Design review of the part built by this model. Coordinates are the model's own, in mm. A direction names the side the tool comes from. Coordinates: 2 decimals unless noted, no trailing zeros. Order: outer loops, then holes, each group sorted by start corner. A loop starts at its lowest first (then second) coordinate and runs counter-clockwise, first axis right, second up. Notation, with made-up numbers: M 73,-16 L 107,-16 A10 cw 107,-5 Z; hole C -39.75,22 d3. An arc over 180 degrees is marked long. Answer in a Markdown table with one row per item.
from build123d import *

# Parameters (mm, degrees)
SKETCH_1_W          = 98
SKETCH_1_H          = 95
EXTRUDE_1_DEPTH     = 1
SKETCH_2_W          = 78
SKETCH_2_H          = 85
EXTRUDE_2_DEPTH     = 20
CUT_EXTRUDE_1_DEPTH = 100
CUT_EXTRUDE_2_DEPTH = 5
SKETCH_5_W          = 9
SKETCH_5_H          = 12
EXTRUDE_3_DEPTH     = 5
SKETCH_6_W          = 11.2
SKETCH_6_H          = 4.6
SKETCH_6_W_2        = 10.2
SKETCH_6_H_2        = 1.749108458
CUT_EXTRUDE_4_DEPTH = 8
CUT_EXTRUDE_5_DEPTH = 0.5


with BuildPart() as part:
    # 스케치1 → 보스-돌출1 (new body)
    with BuildSketch(Plane(origin=(0, 0, 0), x_dir=(1, 0, 0), z_dir=(0, 1, 0))):
        Rectangle(SKETCH_1_W, SKETCH_1_H)
    extrude(amount=EXTRUDE_1_DEPTH)

    # 스케치2 → 보스-돌출2 (add)
    with BuildSketch(Plane(origin=(0, 1, 0), x_dir=(1, 0, 0), z_dir=(0, 1, 0))):
        with Locations((5, 0)):
            Rectangle(SKETCH_2_W, SKETCH_2_H)
    extrude(amount=EXTRUDE_2_DEPTH)

    # 스케치4 → 컷-돌출1 (cut)
    with BuildSketch(Plane(origin=(44, 0, 0), x_dir=(0, 0, -1), z_dir=(1, 0, 0))):
        with BuildLine():
            Line((-42.5, 1), (-41.5, 1))
            Line((-41.5, 1), (-41.5, 12.254740451))
            Line((-41.5, 12.254740451), (-40.591554577, 12.962724137))
            ThreePointArc((-40.591554577, 12.962724137), (-37.80324019, 18.684012014), (-31.875, 21))
            Line((-31.875, 21), (-42.5, 21))
            Line((-42.5, 21), (-42.5, 1))
        make_face()
        with BuildLine():
            Line((-22.25, 12.254740451), (-22.25, 1))
            Line((-22.25, 1), (-20.25, 1))
            Line((-20.25, 1), (-20.25, 12.254740451))
            Line((-20.25, 12.254740451), (-19.341554577, 12.962724137))
            ThreePointArc((-19.341554577, 12.962724137), (-16.553240185, 18.684012019), (-10.624999986, 21))
            Line((-10.624999986, 21), (-31.875, 21))
            ThreePointArc((-31.875, 21), (-25.94675981, 18.684012014), (-23.158445423, 12.962724137))
            Line((-23.158445423, 12.962724137), (-22.25, 12.254740451))
        make_face()
        with BuildLine():
            Line((-1, 12.254740451), (-1, 1))
            Line((-1, 1), (1, 1))
            Line((1, 1), (1, 12.254740451))
            Line((1, 12.254740451), (1.908445423, 12.962724137))
            ThreePointArc((1.908445423, 12.962724137), (4.696759796, 18.684012001), (10.62499996, 21))
            Line((10.62499996, 21), (-10.624999986, 21))
            ThreePointArc((-10.624999986, 21), (-4.696759805, 18.68401201), (-1.908445423, 12.962724137))
            Line((-1.908445423, 12.962724137), (-1, 12.254740451))
        make_face()
        with BuildLine():
            Line((20.25, 12.254740451), (20.25, 1))
            Line((20.25, 1), (22.25, 1))
            Line((22.25, 1), (22.25, 12.254740451))
            Line((22.25, 12.254740451), (23.158445423, 12.962724137))
            ThreePointArc((23.158445423, 12.962724137), (25.94675981, 18.684012014), (31.875, 21))
            Line((31.875, 21), (10.62499996, 21))
            ThreePointArc((10.62499996, 21), (16.553240175, 18.684012028), (19.341554577, 12.962724137))
            Line((19.341554577, 12.962724137), (20.25, 12.254740451))
        make_face()
        with BuildLine():
            Line((42.5, 21), (31.875, 21))
            ThreePointArc((31.875, 21), (37.80324019, 18.684012014), (40.591554577, 12.962724137))
            Line((40.591554577, 12.962724137), (41.5, 12.254740451))
            Line((41.5, 12.254740451), (41.5, 1))
            Line((41.5, 1), (42.5, 1))
            Line((42.5, 1), (42.5, 21))
        make_face()
    extrude(amount=-CUT_EXTRUDE_1_DEPTH, mode=Mode.SUBTRACT)

    # 스케치4<3> → 컷-돌출2 (cut)
    with BuildSketch(Plane(origin=(44, 0, 0), x_dir=(0, 0, -1), z_dir=(1, 0, 0))):
        with BuildLine():
            ThreePointArc((-23.158445423, 12.962724137), (-31.875, 21), (-40.591554577, 12.962724137))
            Line((-40.591554577, 12.962724137), (-36.685, 16.007240451))
            Line((-36.685, 16.007240451), (-27.065, 16.007240451))
            Line((-27.065, 16.007240451), (-23.158445423, 12.962724137))
        make_face()
        with BuildLine():
            Line((-5.815, 16.007240451), (-1.908445423, 12.962724137))
            ThreePointArc((-1.908445423, 12.962724137), (-10.625, 21), (-19.341554577, 12.962724137))
            Line((-19.341554577, 12.962724137), (-15.435, 16.007240451))
            Line((-15.435, 16.007240451), (-5.815, 16.007240451))
        make_face()
        with BuildLine():
            Line((15.435, 16.007240451), (19.341554577, 12.962724137))
            ThreePointArc((19.341554577, 12.962724137), (10.625, 21), (1.908445423, 12.962724137))
            Line((1.908445423, 12.962724137), (5.815, 16.007240451))
            Line((5.815, 16.007240451), (15.435, 16.007240451))
        make_face()
        with BuildLine():
            Line((36.685, 16.007240451), (40.591554577, 12.962724137))
            ThreePointArc((40.591554577, 12.962724137), (31.875, 21), (23.158445423, 12.962724137))
            Line((23.158445423, 12.962724137), (27.065, 16.007240451))
            Line((27.065, 16.007240451), (36.685, 16.007240451))
        make_face()
    extrude(amount=-CUT_EXTRUDE_2_DEPTH, mode=Mode.SUBTRACT)

    # 스케치5 → 보스-돌출3 (add)
    with BuildSketch(Plane(origin=(0, 1, 0), x_dir=(1, 0, 0), z_dir=(0, 1, 0))):
        with Locations((-44.5, 0)):
            Rectangle(SKETCH_5_W, SKETCH_5_H)
    extrude(amount=EXTRUDE_3_DEPTH)

    # 스케치6 → 컷-돌출4 (cut)
    with BuildSketch(Plane.ZY.offset(49)):
        with Locations((0, 3.3)):
            Rectangle(SKETCH_6_W, SKETCH_6_H)
        with Locations((0, 4.300145796)):
            Rectangle(SKETCH_6_W_2, SKETCH_6_H_2, mode=Mode.SUBTRACT)
    extrude(amount=-CUT_EXTRUDE_4_DEPTH, mode=Mode.SUBTRACT)

    # 스케치7 → 컷-돌출5 (cut)
    with BuildSketch(Plane(origin=(0, 6, 0), x_dir=(1, 0, 0), z_dir=(0, 1, 0))):
        Polygon((-42.731367286, 2.836850655), (-46.283445156, 2.836850655), (-47.255371975, 2.487236692), (-47.255371975, 1.305541495), (-46.33938339, 0.68322864), (-42.731367286, 0.68322864), (-42.731367286, 0.994385067), (-46.33938339, 0.994385067), (-46.960091467, 1.416087501), (-46.960091467, 2.396337061), (-46.33938339, 2.619613348), (-42.731367286, 2.619613348), align=None)
        Polygon((-42.731367286, -2.836850655), (-46.283445156, -2.836850655), (-47.255371975, -2.487236692), (-47.255371975, -1.305541495), (-46.33938339, -0.68322864), (-42.731367286, -0.68322864), (-42.731367286, -0.994385067), (-46.33938339, -0.994385067), (-46.960091467, -1.416087501), (-46.960091467, -2.396337061), (-46.33938339, -2.619613348), (-42.731367286, -2.619613348), align=None)
    extrude(amount=-CUT_EXTRUDE_5_DEPTH, mode=Mode.SUBTRACT)


solid = part.part
(1) Draft analysis for pull direction Y (two halves, no side actions). For faces 4 (the flat face through (-34, 11, 32)), 5 (the flat face through (42, 16.007, 32)), 6 (the flat face through (-45, 5.6, 0)), state which applies: pulls with the +Y half, pulls with the -Y half, needs draft (parallel to the pull), parting line crosses it, or undercut.
Return value:
| item | result |
|---|---|
| face 4 | needs draft |
| face 5 | pulls with the +Y half |
| face 6 | undercut |
(2) Insertion check: pin 1 Ø2.5 at (x, z) = (42.5, 11.5) entering from +Y; pin 2 Ø6 at (y, z) = (8, -28.5) entering from -X; pin 3 Ø1.5 at (x, y) = (33, 4) entering from -Z; pin 4 Ø3 at (x, z) = (-39, 13) entering from -Y. Each pin has a flat end and moves straight along its axis. Give the tip position at first contact, or say it passes through.
Return value:
| item | result |
|---|---|
| pin 1 | stops at y = 16.01 |
| pin 2 | stops at x = -34 |
| pin 3 | stops at z = -41.5 |
| pin 4 | stops at y = 0 |
(3) Add section C-C, the plane z = 30.5. Give the boundary of the cut face in (x, y).
Return value:
| item | result |
|---|---|
| outline | M -49,0 L 49,0 L 49,1 L 44,1 L 44,16.01 L 39,16.01 L 39,20.89 L -34,20.89 L -34,1 L -49,1 Z |
(4) For line 1 along Z through (x, y) = (-1.5, 4); line 2 along Z through (x, y) = (-42, 4.75); line 3 along Z through (x, y) = (16, 16.5), list the stretches that pass through material, from the lowest coordinate up. Write a range as from..to.
Return value:
| item | result |
|---|---|
| line 1 | z = -41.5..-22.25, -20.25..-1, 1..20.25, 22.25..41.5 |
| line 2 | z = -6..-5.6, -5.1..5.1, 5.6..6 |
| line 3 | z = -39.52..-24.23, -18.27..-2.98, 2.98..18.27, 24.23..39.52 |
(5) Add section B-B, the plane x = 14.5. Give the boundary of the cut face in (y, z) (3 decimals), and give its area (3 significant figures).
Return value:
| item | result |
|---|---|
| outline | M 0,-47.5 L 1,-47.5 L 1,-41.5 L 12.255,-41.5 L 12.963,-40.592 A8.745 ccw 12.963,-23.158 L 12.255,-22.25 L 1,-22.25 L 1,-20.25 L 12.255,-20.25 L 12.963,-19.342 A8.745 ccw 12.963,-1.908 L 12.255,-1 L 1,-1 L 1,1 L 12.255,1 L 12.963,1.908 A8.745 ccw 12.963,19.342 L 12.255,20.25 L 1,20.25 L 1,22.25 L 12.255,22.25 L 12.963,23.158 A8.745 ccw 12.963,40.592 L 12.255,41.5 L 1,41.5 L 1,47.5 L 0,47.5 Z |
| area | 1,440 mm2 |
(6) Add section D-D, the plane y = 18.25. Give the boundary of the cut face in (x, z).
Return value:
| item | result |
|---|---|
| outline | M -34,-38.24 L 39,-38.24 L 39,-25.51 L -34,-25.51 Z; M -34,-16.99 L 39,-16.99 L 39,-4.26 L -34,-4.26 Z; M -34,4.26 L 39,4.26 L 39,16.99 L -34,16.99 Z; M -34,25.51 L 39,25.51 L 39,38.24 L -34,38.24 Z |
(7) For faces 1 (the flat face through (6, 7, -20.25)), 2 (the flat face through (-45, 3, 5.6)), 3 (the flat face through (6, 7, -41.5)), list the 3-axis set-ups (+Z, -Z, +X, -X, +Y, -Y) from which the entire face can be reached by the end or side of a thin tool; tool diameter is ignored.
Return value:
| item | result |
|---|---|
| face 1 | +X, -X, +Y |
| face 2 | -X |
| face 3 | -Z, +X, -X, +Y |
(8) Add section A-A, the plane y = 10. Give the boundary of the cut face in (x, z), and give its area (3 significant figures).
Return value:
| item | result |
|---|---|
| outline | M -34,-41.5 L 44,-41.5 L 44,-22.25 L -34,-22.25 Z; M -34,-20.25 L 44,-20.25 L 44,-1 L -34,-1 Z; M -34,1 L 44,1 L 44,20.25 L -34,20.25 Z; M -34,22.25 L 44,22.25 L 44,41.5 L -34,41.5 Z |
| area | 6,010 mm2 |
